Geometry: final body of the model. Coordinates: model frame, mm. A direction names the side the tool comes from. Round coordinates to 2 decimals unless told otherwise and drop trailing zeros. Order: outer loops, then holes, each group sorted by start corner. A loop starts at its lowest first (then second) coordinate and runs counter-clockwise, first axis right, second up. Notation, with made-up numbers: M 59.25,24.5 L 115.25,24.5 A20 ccw 115.25,35.5 Z; hole C -16,51 d9. An arc over 180 degrees is marked long. Return JSON: item names as keys, results as strings. Group by question number.
Q1. Cut plane C-C on y = 53. Output: boundary loops of the cut face in (x, z), and give its area (3 significant figures).
Q2. Cut plane A-A on y = 31.75. Output: boundary loops of the cut face in (x, z), and give its area (3 significant figures).
Q3. Access query for faces 4 (the face through (75.844, 29.843, -6.057)), 5 (the face through (15.601, 6.439, -13.765)), 6 (the face through (-50.8, 31, 0)). Directions: +Z, -Z, +X, -X, +Y, -Y. A direction counts if a zero-diameter tool reaches every point of the face in a straight line with its end or side. Return the directions, or none.
Q4. Cut plane D-D on z = -20.5. Output: boundary loops of the cut face in (x, y).
Q5. Cut plane B-B on z = 0. Output: boundary loops of the cut face in (x, y), and give its area (3 significant figures).
Q6. Mould query, pull axis Z, two halves, no side actions, for faces 1 (the face through (101.6, 32, 0)), 2 (the face through (16.936, 13.684, -12.625)), 3 (the face through (1, 31, -31.75)). Classes: released by +Z, released by -Z, zero draft, split by the parting line, or undercut.
Q7. Ray query, probe 1 along X at (y, z) = (10, 12.5); probe 2 along X at (y, z) = (3, 12.7); probe 3 along X at (y, z) = (50.5, -29). Return the intervals inside material, ascending.
Q8. Contact query for flat-ended pins moving along their axis: pin 1 (1 mm diameter, centred on x = 75.5, z = -1.5, fed in from -Y); pin 2 (3 mm diameter, centred on y = 29.5, z = 15.5, fed in from +X). Output: stop coordinate, or through.
Autodesk Inventor part; units mm, degrees
ref_plane "YZ Plane" through (0, 0, 0) normal (1, 0, 0) x (0, 1, 0)
ref_plane "XZ Plane" through (0, 0, 0) normal (0, 1, 0) x (-1, 0, 0)
ref_plane "XY Plane" through (0, 0, 0) normal (0, 0, 1) x (1, 0, 0)
sketch "Sketch1" plane through (0, 0, 0) normal (0, 1, 0) x (-1, 0, 0)
  line L0 (50.8, 31.75) -> (-50.8, 31.75)
  line L1 (-50.8, 31.75) -> (-50.8, -31.75)
  line L2 (-50.8, -31.75) -> (50.8, -31.75)
  line L3 (50.8, -31.75) -> (50.8, 31.75)
  line L4 (50.8, 31.75) -> (-50.8, -31.75) construction
  line L5 (-50.8, 31.75) -> (50.8, -31.75) construction
  point P0 (0, 0)
  dimension "d0" = 101.6
  dimension "d1" = 63.5
extrude "Extrusion1" add sketch "Sketch1" along normal blind 63.5
sketch "Sketch2" plane through (0, 0, 0) normal (0, -1, 0) x (1, 0, 0)
  line L0 (17.272, 12.7) -> (-17.272, 12.7) construction
  line L1 (-17.272, 12.7) -> (-17.272, -12.7) construction
  line L2 (-17.272, -12.7) -> (17.272, -12.7) construction
  line L3 (17.272, -12.7) -> (17.272, 12.7) construction
  line L4 (17.272, 12.7) -> (-17.272, -12.7) construction
  line L5 (-17.272, 12.7) -> (17.272, -12.7) construction
  point P0 (0, 0)
  dimension "d5" = 34.544
  dimension "d6" = 25.4
hole "Hole1" at (17.272, 0, -12.7) at (-17.272, 0, -12.7) at (-17.272, 0, 12.7) at (17.272, 0, 12.7) direction (0, 1, 0) diameter 3.9624 depth 12.7 tip angle 118
sketch "Sketch3" plane through (50.8, 0, 31.75) normal (1, 0, 0) x (0, 0, -1)
  circle A0 centre (31.75, 31.75) radius 6.35
  line L0 (0, 0) -> (0, 63.5)
  line L1 (0, 0) -> (63.5, 0)
  point P0 (31.75, 0)
  dimension "d14" = 12.7
  dimension "d15" = 31.75
  dimension "d16" = 31.75
extrude "Extrusion2" add sketch "Sketch3" along normal blind 50.8
properties part number "BaneBot220GearBox"
Result sheet:
{
 "1": {"outline": "M -50.8,-31.75 L 50.8,-31.75 L 50.8,31.75 L -50.8,31.75 Z", "area": "6,450 mm²"},
 "2": {"outline": "M -50.8,-31.75 L 50.8,-31.75 L 50.8,-6.35 L 101.6,-6.35 L 101.6,6.35 L 50.8,6.35 L 50.8,31.75 L -50.8,31.75 Z", "area": "7,100 mm²"},
 "3": {"face 4": "+X", "face 5": "-Y", "face 6": "+Z, -Z, -X, +Y, -Y"},
 "4": {"outline": "M -50.8,0 L 50.8,0 L 50.8,63.5 L -50.8,63.5 Z"},
 "5": {"outline": "M -50.8,0 L 50.8,0 L 50.8,25.4 L 101.6,25.4 L 101.6,38.1 L 50.8,38.1 L 50.8,63.5 L -50.8,63.5 Z", "area": "7,100 mm²"},
 "6": {"face 1": "zero draft", "face 2": "undercut", "face 3": "released by -Z"},
 "7": {"probe 1": "x = -50.8 to -19.24, -15.3 to 15.3, 19.24 to 50.8", "probe 2": "x = -50.8 to -19.25, -15.29 to 15.29, 19.25 to 50.8", "probe 3": "x = -50.8 to 50.8"},
 "8": {"pin 1": "stops at y = 25.48", "pin 2": "stops at x = 50.8"}
}
